```python
from build123d import *

# Parameters (mm, degrees)
BOSS_EXTRUDE1_DEPTH                        = 10
CBORE_FOR_M4_CHEESE_HEAD_SCREW1_AT_2_COUNT = 2
CBORE_FOR_M4_CHEESE_HEAD_SCREW1_AT_2_PITCH = 114
SKETCH6_R                                  = 4
CUT_EXTRUDE1_DEPTH                         = 8


with BuildPart() as part:
    # Sketch1 → Boss-Extrude1 (new body)
    with BuildSketch(Plane(origin=(0, 0, 0), x_dir=(0, 0, -1), z_dir=(1, 0, 0))):
        with BuildLine():
            Line((30, 49.547642934), (30, 54.216993929))
            ThreePointArc((30, 54.216993929), (29.713903717, 55.237294084), (28.93903477, 55.960095305))
            ThreePointArc((28.93903477, 55.960095305), (0, 63), (-28.93903477, 55.960095305))
            ThreePointArc((-28.93903477, 55.960095305), (-29.713903717, 55.237294084), (-30, 54.216993929))
            Line((-30, 54.216993929), (-30, 49.547642934))
            ThreePointArc((-30, 49.547642934), (-30.239236403, 48.608646152), (-30.898614566, 47.898597244))
            ThreePointArc((-30.898614566, 47.898597244), (-44.936698638, 35.066980416), (-53.971882891, 18.331280838))
            ThreePointArc((-53.971882891, 18.331280838), (-54.687108259, 17.367169566), (-55.830018745, 17))
            Line((-55.830018745, 17), (-60.037612586, 17))
            ThreePointArc((-60.037612586, 17), (-61.425230034, 16.425230034), (-62, 15.037612586))
            Line((-62, 15.037612586), (-62, 2))
            Line((-62, 2), (-51.961524227, 2))
            ThreePointArc((-51.961524227, 2), (0, 52), (51.961524227, 2))
            Line((51.961524227, 2), (62, 2))
            Line((62, 2), (62, 15.037612586))
            ThreePointArc((62, 15.037612586), (61.425230034, 16.425230034), (60.037612586, 17))
            Line((60.037612586, 17), (55.830018745, 17))
            ThreePointArc((55.830018745, 17), (54.687108259, 17.367169566), (53.971882891, 18.331280838))
            ThreePointArc((53.971882891, 18.331280838), (44.936698638, 35.066980416), (30.898614566, 47.898597244))
            ThreePointArc((30.898614566, 47.898597244), (30.239236403, 48.608646152), (30, 49.547642934))
        make_face()
    extrude(amount=BOSS_EXTRUDE1_DEPTH)

    # Sketch4 → CBORE for M4 Cheese Head Screw1 (revolve, cut)
    with BuildSketch(Plane(origin=(5, 17, -57), x_dir=(0, 0, 1), z_dir=(1, 0, 0))):
        Polygon((0, 0), (0, 21.291850331), (2.15, 20), (2.15, 6.6), (4, 6.6), (4, 0), align=None)
    cbore_for_m4_cheese_head_screw1 = revolve(axis=Axis((5, 23.35, -57), (0, -1, 0)), mode=Mode.SUBTRACT)

    # CBORE for M4 Cheese Head Screw1 at 2: CBORE for M4 Cheese Head Screw1 ×2
    with Locations(*[(0, 0, i * CBORE_FOR_M4_CHEESE_HEAD_SCREW1_AT_2_PITCH) for i in range(1, CBORE_FOR_M4_CHEESE_HEAD_SCREW1_AT_2_COUNT)]):
        add(cbore_for_m4_cheese_head_screw1, mode=Mode.SUBTRACT)

    # Sketch6 → Cut-Extrude1 (cut)
    with BuildSketch(Plane(origin=(0, 17, 0), x_dir=(1, 0, 0), z_dir=(0, 1, 0))):
        with Locations((5, 57)):
            Circle(SKETCH6_R)
        with Locations((5, -57)):
            Circle(SKETCH6_R)
    extrude(amount=CUT_EXTRUDE1_DEPTH, mode=Mode.SUBTRACT)


solid = part.part
```
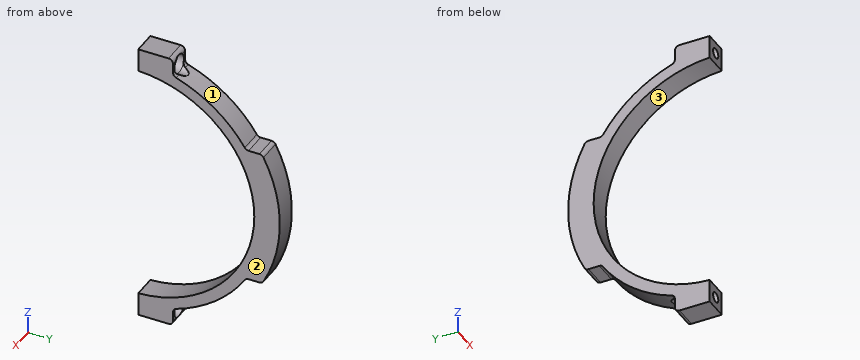
Input: part model. Units: mm. Frame: model coordinates. Face numbers are marked on the shaded views. Round coordinates to 2 decimals unless told otherwise and drop trailing zeros. Loops run counter-clockwise (first coordinate to the right, second up) from the corner with the lowest first, then second, coordinate; pieces in that order, holes last. Notation, with made-up numbers: (38, -6.75) - (45, -6.75) arc R27 cw to (45, 11.25) - close; hole circle Ø4 at (4, 39). An arc over 180 degrees is marked (long way). One line per item, written item: value. Start each with the question number.
(1) Ray query, line 1 (X direction, y = 12, z = 57); line 2 (X direction, y = 4.25, z = -57); line 3 (Z direction, x = 5, y = 8). Return the intervals inside material, ascending. Write a range as [from, to].
(2) Section D-D, the plane y = 30. Return loops of the section in (x, z), plus the area to 3 significant figures.
(3) Contact query for flat-ended pins moving along their axis: P1, Ø1.9, axis at x = 1.5, z = -57.5, coming from the +Y side; P2, Ø1.4, axis at x = 6, y = 53, coming from the -Z side; P3, Ø5, axis at x = 8.5, z = -30, coming from the +Y side. Output: stop coordinate, or through.
(4) Section C-C, the plane x = 5. Count the separate pieces of the cut face and the enclosed holes in it, plus the area to 3 significant figures.
(5) Draft query along Z for the marked faces 1, 2 and 3. Return one class per face: +Z half, -Z half, draft (parallel to the pull), parting line (faces both ways), or undercut.
(6) Section B-B, the plane y = 8. Return loops of the section in (x, z), plus the area to 3 significant figures.
(7) Section A-A, the plane z = -57. Return loops of the section in (x, y), plus the area to 3 significant figures.
Results below:
1. line 1: [0, 1], [9, 10]
1. line 2: [0, 2.85], [7.15, 10]
1. line 3: [-62, -59.15], [-54.85, -51.38], [51.38, 54.85], [59.15, 62]
2. outline: (0, -48.47) - (10, -48.47) - (10, -42.47) - (0, -42.47) - close; (0, 42.47) - (10, 42.47) - (10, 48.47) - (0, 48.47) - close
2. area: 120 mm^2
3. P1: y = 17
3. P2: z = -30
3. P3: y = 56.68
4. separate pieces: 3
4. enclosed holes: 0
4. area: 1,210 mm^2
5. face 1: +Z half
5. face 2: draft
5. face 3: undercut
6. outline: (0, -62) - (10, -62) - (10, -51.38) - (0, -51.38) - close; (0, 51.38) - (10, 51.38) - (10, 62) - (0, 62) - close; hole circle Ø4.3 at (5, -57); hole circle Ø4.3 at (5, 57)
6. area: 183 mm^2
7. outline: (0, 2) - (2.85, 2) - (2.85, 10.4) - (1, 10.4) - (1, 17) - (0, 17) - close; (7.15, 2) - (10, 2) - (10, 17) - (9, 17) - (9, 10.4) - (7.15, 10.4) - close
7. area: 61.1 mm^2
